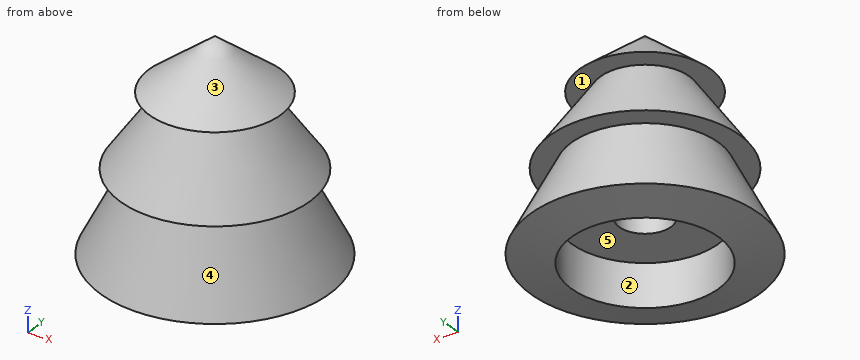
```python
from build123d import *

# Parameters (mm, degrees)
F1_FACE_R = 32.501076
F2_DEPTH  = 25.4
F3_R      = 11.43
F4_DEPTH  = 84.328


with BuildPart() as f1:
    # F0 (on Front) → F1 (revolve)
    with BuildSketch(Plane.XZ):
        Polygon((0, -50.117204), (0, 51.482796), (-28.950538, 27.994625), (-19.664516, 27.994625), (-41.787097, -3.960215), (-32.501076, -3.960215), (-50.526883, -39.738708), (-32.501076, -43.562369), (-32.501076, -50.117204), align=None)
    revolve(axis=Axis((0, 0, 0.682796), (0, 0, 1)))

    # F1_face (on face) → F2 (cut)
    with BuildSketch(Plane(origin=(0, 0, -50.117204), x_dir=(1, 0, 0), z_dir=(0, 0, -1))):
        Circle(F1_FACE_R)
    extrude(amount=-F2_DEPTH, mode=Mode.SUBTRACT)

    # F3 (on Top) → F4 (cut)
    with BuildSketch(Plane.XY):
        Circle(F3_R)
    extrude(amount=-F4_DEPTH, mode=Mode.SUBTRACT)


solid = f1.part
```
Work out the finished part from the listing and answer in its coordinate system (mm). Face numbers are marked on the shaded views. A direction names the side the tool comes from. Round coordinates to 2 decimals unless told otherwise and drop trailing zeros. Loops run counter-clockwise (first coordinate to the right, second up) from the corner with the lowest first, then second, coordinate; pieces in that order, holes last. Notation, with made-up numbers: (38, 56) -> (79, 56) arc R17 ccw to (79, 67) -> close; hole circle Ø2 at (-28, 13). An arc over 180 degrees is marked (long way). Write each question's results on one line, items separated by ' | '. Start each with the question number.
1. For a pull along Z with two mould halves and no side action, classify the marked faces 1, 2 and 3 as +Z half, -Z half, draft (parallel to the pull), parting line (faces both ways), or undercut.
2. Section D-D (z = 3) is taken. Determine the outline of the cut face in (x, y), plus the area to 3 significant figures.
3. Given pin 1 Ø3 at (x, y) = (16, -19.5) entering from +Z (3 decimals); pin 2 Ø25 at (x, y) = (0.5, -20.5) entering from -Z; pin 3 Ø7 at (x, y) = (2.5, 0.5) entering from -Z; pin 4 Ø10 at (x, y) = (-31, -20.5) entering from +Z, each flat-ended and moving along its own axis, determine where each tip first touches the part or whether it passes through.
4. Section B-B (z = 42.5) is taken. Determine the outline of the cut face in (x, y), plus the area to 3 significant figures.
5. Section C-C (z = -9) is taken. Determine the outline of the cut face in (x, y).
6. Find the intervals of material crossed by probe 1 along Y at (x, z) = (0, -8.5); probe 2 along X at (y, z) = (0, -36); probe 3 along Y at (x, z) = (0, -14), in increasing order. Write a range as from..to.
7. A tool of negligible diameter and unlimited length cuts with its end or side. For the marked faces 4 and 5, from which of +Z, -Z, +X, -X, +Y, -Y can it reach the whole face along a straight path? Write none if from no direction.
8. Section A-A (z = -29.5) is taken. Determine the outline of the cut face in (x, y), plus the area to 3 significant figures.
Evaluation:
1) face 1: undercut | face 2: draft | face 3: +Z half
2) outline: circle Ø73.94 at (0, 0) | area: 4,290 mm2
3) pin 1: stops at z = 32.235 | pin 2: stops at z = -43.56 | pin 3: stops at z = 0 | pin 4: stops at z = 9.94
4) outline: circle Ø22.14 at (0, 0) | area: 385 mm2
5) outline: circle Ø70.08 at (0, 0); hole circle Ø22.86 at (0, 0)
6) probe 1: y = -34.79..-11.43, 11.43..34.79 | probe 2: x = -48.64..-32.5, 32.5..48.64 | probe 3: y = -37.56..-11.43, 11.43..37.56
7) face 4: none | face 5: -Z
8) outline: circle Ø90.74 at (0, 0); hole circle Ø65 at (0, 0) | area: 3,150 mm2
